Check sheet for the modelled part. Datum: model origin and axes. Units: mm. Face numbers are marked on the shaded views. Coordinates: 2 decimals unless noted, no trailing zeros. Order: outer loops, then holes, each group sorted by start corner. A loop starts at its lowest first (then second) coordinate and runs counter-clockwise, first axis right, second up.
1. Cross-section at C-C (y = 36.5). Enter the section's corners in (x, z).
2. Cross-section at D-D (y = 15.5). Enter the section's corners in (x, z).
3. Thickness scan on line 1 (Y direction, x = 97.5, z = 8); line 2 (X direction, y = 5.5, z = 5.25); line 3 (X direction, y = 32.5, z = 9). Record the ranges inside material, lowest first.
4. Draft check along X on the marked faces 1, 2 and 3. Enter one of: released by +X, released by -X, zero draft, split by the parting line, or undercut.
5. Gauge pin test, flat ends, axial feed: pin 1 Ø5 at (y, z) = (33.5, 6) entering from -X; pin 2 Ø4 at (x, y) = (14, 5.5) entering from -Z; pin 3 Ø3 at (x, z) = (56, 5) entering from +Y; pin 4 Ø2 at (y, z) = (76, 1.5) entering from -X. Record the tip position at first contact, or that the pin passes through.
6. Cross-section at A-A (x = 76). Enter the section's corners in (y, z), then the cut area to 3 significant figures.
7. Cross-section at B-B (y = 55.5). Enter the section's corners in (x, z), then the cut area to 3 significant figures.
```python
from build123d import *

# Parameters (mm, degrees)
BOSS_EXTRUDE1_DEPTH                      = 10
FILLET1_R                                = 5
FILLET2_R                                = 10
SKETCH2_R                                = 9
CUT_EXTRUDE1_DEPTH                       = 177.171081622
SKETCH3_R                                = 6.5
CUT_EXTRUDE2_DEPTH                       = 177.171081622
SKETCH4_W                                = 46
SKETCH4_H                                = 46
CUT_EXTRUDE3_DEPTH                       = 177.171081622
CUT_EXTRUDE4_REACH                       = 178.171
CUT_EXTRUDE4_END_RADIUS                  = 9
SKETCH5_R                                = 1.5
FILLET3_R                                = 5
M3X0_5_TAPPED_HOLE1_D                    = 2.6
M3X0_5_TAPPED_HOLE1_DEPTH                = 9
M3X0_5_TAPPED_HOLE1_TIP                  = 0.781118805
CBORE_FOR_M3_PAN_HEAD_SCREW1_D           = 3.4
CBORE_FOR_M3_PAN_HEAD_SCREW1_CBORE_D     = 6.5
CBORE_FOR_M3_PAN_HEAD_SCREW1_CBORE_DEPTH = 3.3
CBORE_FOR_M3_PAN_HEAD_SCREW2_D           = 3.4
CBORE_FOR_M3_PAN_HEAD_SCREW2_CBORE_D     = 6.5
CBORE_FOR_M3_PAN_HEAD_SCREW2_CBORE_DEPTH = 3.3


with BuildPart() as part:
    # Sketch1 → Boss-Extrude1 (new body)
    with BuildSketch(Plane.XY):
        with BuildLine():
            Line((0, 0), (152, 0))
            Line((152, 0), (152, 76))
            Line((152, 76), (65.450849719, 76))
            ThreePointArc((65.450849719, 76), (24.119171634, 86.031463461), (0, 51))
            Line((0, 51), (0, 0))
        make_face()
    extrude(amount=BOSS_EXTRUDE1_DEPTH)

    # Fillet1
    fillet1_edges = [part.edges().sort_by_distance(p)[0] for p in [
        (65.450849719, 76, 5),
    ]]
    fillet(fillet1_edges, radius=FILLET1_R)

    # Fillet2
    fillet2_edges = [part.edges().sort_by_distance(p)[0] for p in [
        (152, 76, 5),
    ]]
    fillet(fillet2_edges, radius=FILLET2_R)

    # Sketch2 → Cut-Extrude1 (cut, through all)
    with BuildSketch(Plane.XY.offset(10)):
        with Locations((37.5, 21)):
            Circle(SKETCH2_R)
    extrude(amount=-CUT_EXTRUDE1_DEPTH, mode=Mode.SUBTRACT)

    # Sketch3 → Cut-Extrude2 (cut, through all)
    with BuildSketch(Plane.XY.offset(10)):
        with Locations((37.5, 51)):
            Circle(SKETCH3_R)
    extrude(amount=-CUT_EXTRUDE2_DEPTH, mode=Mode.SUBTRACT)

    # Sketch4 → Cut-Extrude3 (cut, through all)
    with BuildSketch(Plane.XY.offset(10)):
        with Locations((85.5, 43)):
            Rectangle(SKETCH4_W, SKETCH4_H)
    extrude(amount=-CUT_EXTRUDE3_DEPTH, mode=Mode.SUBTRACT)

    # Cut-Extrude4: up to this cylinder (the profile starts outside it)
    cut_extrude4_end = Plane(origin=(37.5, 21, 2.5), z_dir=(0, 0, 1)) * Cylinder(CUT_EXTRUDE4_END_RADIUS, 375.342, mode=Mode.PRIVATE)
    # Sketch5 → Cut-Extrude4 (cut, up to the surface)
    with BuildSketch(Plane.XZ, mode=Mode.PRIVATE) as cut_extrude4_sk1:
        with Locations(Location((37.5, 2.5, 0), (0, 0, 270))):
            Circle(SKETCH5_R)
    cut_extrude4_tool1 = extrude(cut_extrude4_sk1.sketch, amount=-CUT_EXTRUDE4_REACH, mode=Mode.PRIVATE) - cut_extrude4_end
    add(cut_extrude4_tool1.solids().sort_by_distance((37.5, 0, 2.5))[0], mode=Mode.SUBTRACT)

    # Fillet3
    fillet3_edges = [part.edges().sort_by_distance(p)[0] for p in [
        (62.5, 20, 5),
        (62.5, 66, 5),
        (108.5, 66, 5),
        (108.5, 20, 5),
    ]]
    fillet(fillet3_edges, radius=FILLET3_R)

    # M3x0.5 Tapped Hole1
    with Locations(Plane(origin=(0, 0, 0), x_dir=(-1, 0, 0), z_dir=(0, -1, 0))):
        with Locations((-16, -5), (-56, -5), (-96, -5), (-136, -5)):
            Hole(M3X0_5_TAPPED_HOLE1_D / 2, depth=M3X0_5_TAPPED_HOLE1_DEPTH)
            with Locations((0, 0, -(M3X0_5_TAPPED_HOLE1_DEPTH + M3X0_5_TAPPED_HOLE1_TIP / 2))):  # 118° drill point
                Cone(0, M3X0_5_TAPPED_HOLE1_D / 2, M3X0_5_TAPPED_HOLE1_TIP, mode=Mode.SUBTRACT)

    # CBORE for M3 Pan Head Screw1 (through all)
    with Locations(Plane(origin=(0, 0, 0), x_dir=(1, 0, 0), z_dir=(0, 0, -1))):
        with Locations((14, -36.5), (45, -36.5), (45, -5.5), (14, -5.5)):
            CounterBoreHole(CBORE_FOR_M3_PAN_HEAD_SCREW1_D / 2, CBORE_FOR_M3_PAN_HEAD_SCREW1_CBORE_D / 2, CBORE_FOR_M3_PAN_HEAD_SCREW1_CBORE_DEPTH)

    # CBORE for M3 Pan Head Screw2 (through all)
    with Locations(Plane(origin=(0, 0, 10), x_dir=(-1, 0, 0), z_dir=(0, 0, 1))):
        with Locations((-127.5, -71), (-102.5, -71)):
            CounterBoreHole(CBORE_FOR_M3_PAN_HEAD_SCREW2_D / 2, CBORE_FOR_M3_PAN_HEAD_SCREW2_CBORE_D / 2, CBORE_FOR_M3_PAN_HEAD_SCREW2_CBORE_DEPTH)


solid = part.part
```
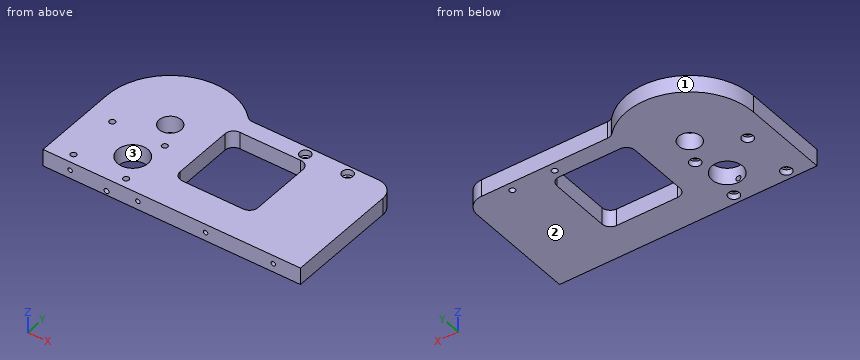
Data:
1. outline: (0, 0) - (10.75, 0) - (10.75, 3.3) - (12.3, 3.3) - (12.3, 10) - (0, 10) - close; (15.7, 3.3) - (17.25, 3.3) - (17.25, 0) - (41.75, 0) - (41.75, 3.3) - (43.3, 3.3) - (43.3, 10) - (15.7, 10) - close; (46.7, 3.3) - (48.25, 3.3) - (48.25, 0) - (62.5, 0) - (62.5, 10) - (46.7, 10) - close; (108.5, 0) - (152, 0) - (152, 10) - (108.5, 10) - close
2. outline: (0, 0) - (30.38, 0) - (30.38, 10) - (0, 10) - close; (44.62, 0) - (152, 0) - (152, 10) - (44.62, 10) - close
3. line 1: y = 0 to 20, 66 to 76
3. line 2: x = 0 to 12.3, 17.28 to 43.3, 46.7 to 54.72, 57.28 to 94.72, 97.28 to 134.72, 137.28 to 152
3. line 3: x = 0 to 62.5, 108.5 to 152
4. face 1: split by the parting line
4. face 2: zero draft
4. face 3: undercut
5. pin 1: stops at x = 0
5. pin 2: stops at z = 3.3
5. pin 3: stops at y = 84.43
5. pin 4: stops at x = 8.69
6. outline: (0, 0) - (20, 0) - (20, 10) - (0, 10) - close; (66, 0) - (76, 0) - (76, 10) - (66, 10) - close
6. area: 300 mm2
7. outline: (0.27, 0) - (32.81, 0) - (32.81, 10) - (0.27, 10) - close; (42.19, 0) - (62.5, 0) - (62.5, 10) - (42.19, 10) - close; (108.5, 0) - (152, 0) - (152, 10) - (108.5, 10) - close
7. area: 963 mm2
